For this review, use the dimensioned drawing (mm, ordinates from the lowest corner) and the shaded views. A direction names the side the tool comes from. Give positions to 0.01 mm unless a question says otherwise; leave off trailing zeros. Order: outer loops, then holes, each group sorted by start corner. A loop starts at its lowest first (then second) coordinate and runs counter-clockwise, first axis right, second up. Notation, with made-up numbers: (-39, 10.25) -> (-4, 10.25) arc R15 cw to (-4, 26.25) -> close; hole circle Ø7 at (44.5, 70.25). An arc over 180 degrees is marked (long way). Return JSON: item names as keys, results as strings.
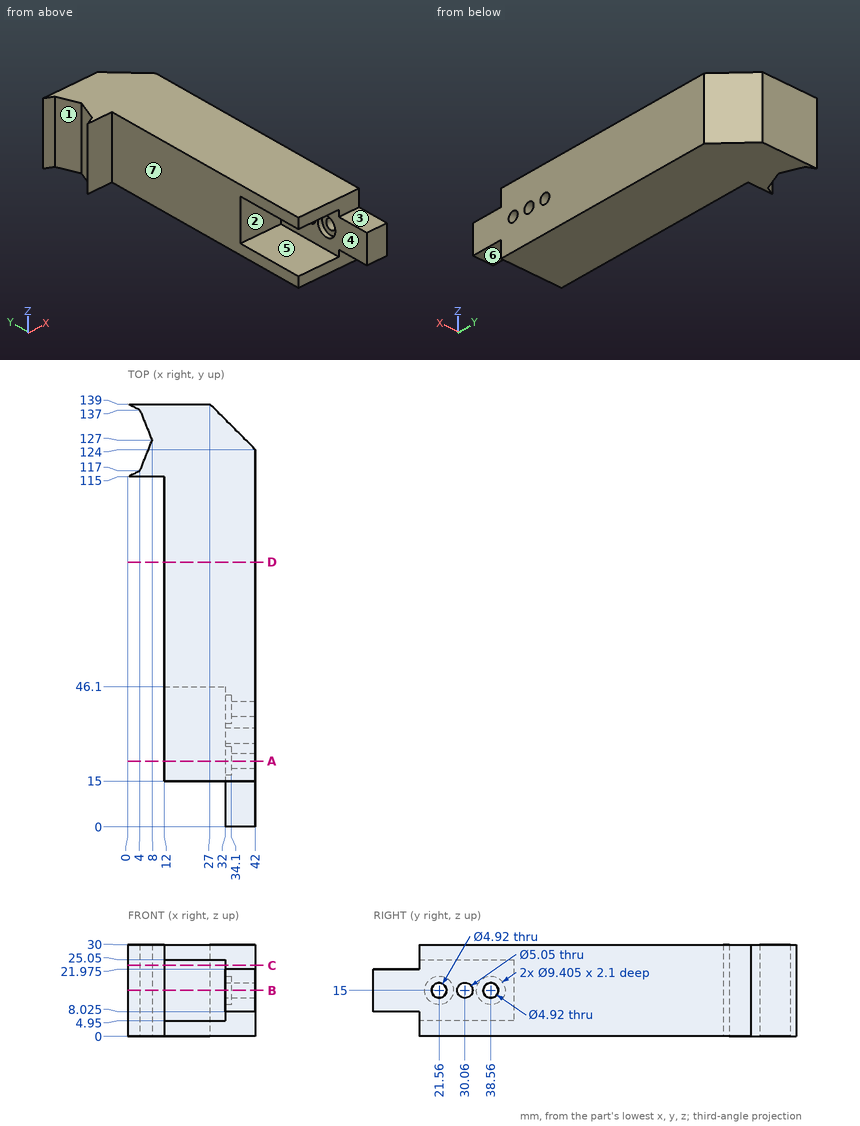
Item 1: Machinability: for the marked faces 1, 2 and 3, which of the approach directions +Z, -Z, +X, -X, +Y, -Y give a long, thin tool a straight path to every point of the face, cutting with its end or side? Answer none if there is none.
Result set:
{"face 1": "+Z, -Z, -X", "face 2": "-X, -Y", "face 3": "+Z, +X, -X, -Y"}
Item 2: For pin 1 (6.5 mm diameter, centred on y = 21.56, z = 15, fed in from -X); pin 2 (10 mm diameter, centred on x = 22.5, z = 14, fed in from -Y); pin 3 (12 mm diameter, centred on y = 21.56, z = 15, fed in from -X), all flat-tipped, find the tip position at first contact; note any pin that passes through.
Result set:
{"pin 1": "stops at x = 34.1", "pin 2": "stops at y = 46.1", "pin 3": "stops at x = 32"}
Item 3: Add section C-C (z = 23.25). Give the boundary of the cut face in (x, y), plus the area to 3 significant figures.
Result set:
{"outline": "(0, 115) -> (12, 115) -> (12, 46.1) -> (32, 46.1) -> (32, 15) -> (42, 15) -> (42, 124) -> (27, 139) -> (0, 139) -> (4, 137) -> (8, 127) -> (4, 117) -> close", "area": "3,150 mm^2"}
Item 4: Add section B-B (z = 15). Give the number of separate pieces and of enclosed holes in the cut face, plus the area to 3 significant figures.
Result set:
{"separate pieces": "4", "enclosed holes": "0", "area": "3,130 mm^2"}
Item 5: Add section A-A (y = 21.56). Give the boundary of the cut face in (x, z), plus the area to 3 significant figures.
Result set:
{"outline": "(12, 0) -> (42, 0) -> (42, 12.54) -> (34.1, 12.54) -> (34.1, 10.3) -> (32, 10.3) -> (32, 4.95) -> (12, 4.95) -> close; (12, 25.05) -> (32, 25.05) -> (32, 19.7) -> (34.1, 19.7) -> (34.1, 17.46) -> (42, 17.46) -> (42, 30) -> (12, 30) -> close", "area": "439 mm^2"}
Item 6: Wall thickness on L1, parallel to Y at x = 36.5, z = 15 (3 decimals); L2, parallel to Y at x = 33, z = 15 (1 decimal); L3, parallel to X at y = 89, z = 18: over which ranges is each line inside the solid? List them lowest first. Write a range as [from, to].
Result set:
{"L1": "y = [0, 19.1], [24.02, 27.535], [32.585, 36.1], [41.02, 129.5]", "L2": "y = [0, 16.9], [26.3, 27.5], [32.6, 33.9], [43.3, 133]", "L3": "x = [12, 42]"}
Item 7: Add section D-D (y = 87). Give the boundary of the cut face in (x, z).
Result set:
{"outline": "(12, 0) -> (42, 0) -> (42, 30) -> (12, 30) -> close"}
Item 8: Mouldability with a two-part tool opening along Z and no side actions: class the marked faces 4, 5, 6 and 7 as released by +Z, released by -Z, zero draft, split by the parting line, or undercut.
Result set:
{"face 4": "undercut", "face 5": "undercut", "face 6": "released by -Z", "face 7": "zero draft"}
